Here's how the part is built. I have some questions about the finished solid (model axes, mm). Face numbers are marked on the shaded views. A direction names the side the tool comes from. Round coordinates to 2 decimals unless told otherwise and drop trailing zeros. Order: outer loops, then holes, each group sorted by start corner. A loop starts at its lowest first (then second) coordinate and runs counter-clockwise, first axis right, second up.
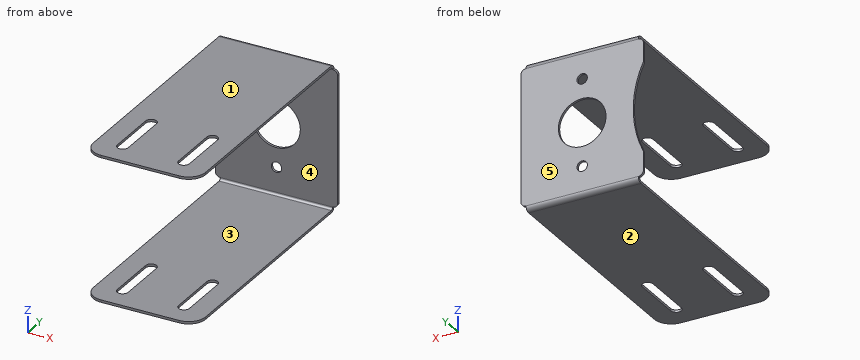
```python
from build123d import *

# Parameters (mm, degrees)
SKETCH1_W               = 36
SKETCH1_H               = 40
BASE_FLANGE1_DEPTH      = 0.7
EDGE_FLANGE1_DEPTH      = 33
EDGE_FLANGE1_BEND_DEPTH = 33
BREAK_CORNER1_START     = -0.7
BREAK_CORNER1_DEPTH     = 0.7
BREAK_CORNER2_START     = -21.4
BREAK_CORNER2_DEPTH     = 42.8
CUT_EXTRUDE1_DEPTH      = 78.892554201
CUT_EXTRUDE1_DEPTH_BACK = 78.892554201
CUT_EXTRUDE2_REACH      = 79.893
SKETCH11_R              = 7
SKETCH11_R_2            = 1.525
CUT_EXTRUDE3_REACH      = 79.893
SKETCH12_R              = 30


# Read off the part's stored shape, not the designer's step: Break-Corner1, Break-Corner2
# Sheet-metal steps are written as plain solids
with BuildPart() as part:
    # Sketch1 → Base-Flange1 (new body)
    with BuildSketch(Plane(origin=(0, 0, 0), x_dir=(1, 0, 0), z_dir=(0, 1, 0))):
        Rectangle(SKETCH1_W, SKETCH1_H)
    extrude(amount=-BASE_FLANGE1_DEPTH)

    # Edge-Flange1 section (across the edge) → Edge-Flange1 (add)
    with BuildSketch(Plane(origin=(16.5, -0.7, 20.7), x_dir=(0, 0, -1), z_dir=(-1, 0, 0))):
        with BuildLine():
            Line((-0.7, 0.7), (-0.7, 72))
            Line((-0.7, 72), (0, 72))
            Line((0, 72), (0, 0.7))
            ThreePointArc((0, 0.7), (0.205025253, 0.205025253), (0.7, 0))
            Line((0.7, 0), (0.7, -0.7))
            ThreePointArc((0.7, -0.7), (-0.289949494, -0.289949494), (-0.7, 0.7))
        make_face()
    extrude(amount=EDGE_FLANGE1_DEPTH)

    # Edge-Flange1 section 2 (across the edge) → Edge-Flange1 bend (add)
    with BuildSketch(Plane(origin=(-16.5, -0.7, -20.7), x_dir=(0, 0, 1), z_dir=(1, 0, 0))):
        with BuildLine():
            Line((-0.7, 0.7), (-0.7, 72))
            Line((-0.7, 72), (0, 72))
            Line((0, 72), (0, 0.7))
            ThreePointArc((0, 0.7), (0.205025253, 0.205025253), (0.7, 0))
            Line((0.7, 0), (0.7, -0.7))
            ThreePointArc((0.7, -0.7), (-0.289949494, -0.289949494), (-0.7, 0.7))
        make_face()
    extrude(amount=EDGE_FLANGE1_BEND_DEPTH)

    # Break-Corner1 outline → Break-Corner1 (cut)
    with BuildSketch(Plane(origin=(0, 0, 0), x_dir=(1, 0, 0), z_dir=(0, 1, 0)).offset(BREAK_CORNER1_START)):
        with BuildLine():
            Line((18, -20), (18, -18.5001))
            ThreePointArc((18, -18.5001), (17.560689461, -19.560689461), (16.5001, -20))
            Line((16.5001, -20), (18, -20))
        make_face()
        with BuildLine():
            ThreePointArc((16.5001, 20), (17.560689461, 19.560689461), (18, 18.5001))
            Line((18, 18.5001), (18, 20))
            Line((18, 20), (16.5001, 20))
        make_face()
        with BuildLine():
            ThreePointArc((-16.5001, -20), (-17.560689461, -19.560689461), (-18, -18.5001))
            Line((-18, -18.5001), (-18, -20))
            Line((-18, -20), (-16.5001, -20))
        make_face()
        with BuildLine():
            ThreePointArc((-18, 18.5001), (-17.560689461, 19.560689461), (-16.5001, 20))
            Line((-16.5001, 20), (-18, 20))
            Line((-18, 20), (-18, 18.5001))
        make_face()
    extrude(amount=BREAK_CORNER1_DEPTH, mode=Mode.SUBTRACT)

    # Break-Corner2 outline → Break-Corner2 (cut)
    with BuildSketch(Plane.XY.offset(BREAK_CORNER2_START)):
        with BuildLine():
            ThreePointArc((16.5, -67.7), (15.035533906, -71.235533906), (11.5, -72.7))
            Line((11.5, -72.7), (16.5, -72.7))
            Line((16.5, -72.7), (16.5, -67.7))
        make_face()
        with BuildLine():
            Line((-16.5, -72.7), (-11.5, -72.7))
            ThreePointArc((-11.5, -72.7), (-15.035533906, -71.235533906), (-16.5, -67.7))
            Line((-16.5, -67.7), (-16.5, -72.7))
        make_face()
    extrude(amount=BREAK_CORNER2_DEPTH, mode=Mode.SUBTRACT)

    # Sketch10 → Cut-Extrude1 (cut, two sides: drawn at the far end of the back side and taken through both)
    with BuildSketch(Plane.XY.offset(-CUT_EXTRUDE1_DEPTH_BACK)):
        with BuildLine():
            Line((-7.4, -50.7), (-7.4, -65.7))
            ThreePointArc((-7.4, -65.7), (-9, -67.3), (-10.6, -65.7))
            Line((-10.6, -65.7), (-10.6, -50.7))
            ThreePointArc((-10.6, -50.7), (-9, -49.1), (-7.4, -50.7))
        make_face()
        with BuildLine():
            Line((7.4, -50.7), (7.4, -65.7))
            ThreePointArc((7.4, -65.7), (9, -67.3), (10.6, -65.7))
            Line((10.6, -65.7), (10.6, -50.7))
            ThreePointArc((10.6, -50.7), (9, -49.1), (7.4, -50.7))
        make_face()
    extrude(amount=CUT_EXTRUDE1_DEPTH + CUT_EXTRUDE1_DEPTH_BACK, mode=Mode.SUBTRACT)

    # Sketch11 → Cut-Extrude2 (cut, up to next)
    with BuildSketch(Plane(origin=(0, 0, 0), x_dir=(1, 0, 0), z_dir=(0, 1, 0)), mode=Mode.PRIVATE) as cut_extrude2_sk1:
        with Locations(Location((0, 0, 0), (0, 0, 270))):
            Circle(SKETCH11_R)
    cut_extrude2_tool1 = extrude(cut_extrude2_sk1.sketch, amount=-CUT_EXTRUDE2_REACH, mode=Mode.PRIVATE) & part.part
    # Sketch11 → Cut-Extrude2 (cut, up to next)
    with BuildSketch(Plane(origin=(0, 0, 0), x_dir=(1, 0, 0), z_dir=(0, 1, 0)), mode=Mode.PRIVATE) as cut_extrude2_sk2:
        with Locations(Location((0, -12.7, 0), (0, 0, 270))):
            Circle(SKETCH11_R_2)
    cut_extrude2_tool2 = extrude(cut_extrude2_sk2.sketch, amount=-CUT_EXTRUDE2_REACH, mode=Mode.PRIVATE) & part.part
    # Sketch11 → Cut-Extrude2 (cut, up to next)
    with BuildSketch(Plane(origin=(0, 0, 0), x_dir=(1, 0, 0), z_dir=(0, 1, 0)), mode=Mode.PRIVATE) as cut_extrude2_sk3:
        with Locations(Location((0, 12.7, 0), (0, 0, 270))):
            Circle(SKETCH11_R_2)
    cut_extrude2_tool3 = extrude(cut_extrude2_sk3.sketch, amount=-CUT_EXTRUDE2_REACH, mode=Mode.PRIVATE) & part.part
    add(cut_extrude2_tool1.solids().sort_by_distance((0, 0, 0))[0], mode=Mode.SUBTRACT)
    add(cut_extrude2_tool2.solids().sort_by_distance((0, 0, 12.7))[0], mode=Mode.SUBTRACT)
    add(cut_extrude2_tool3.solids().sort_by_distance((0, 0, -12.7))[0], mode=Mode.SUBTRACT)

    # Sketch12 → Cut-Extrude3 (cut, up to next)
    with BuildSketch(Plane(origin=(0, 0, 0), x_dir=(1, 0, 0), z_dir=(0, 1, 0)), mode=Mode.PRIVATE) as cut_extrude3_sk1:
        with Locations((-45, 0)):
            Circle(SKETCH12_R)
    cut_extrude3_tool1 = extrude(cut_extrude3_sk1.sketch, amount=-CUT_EXTRUDE3_REACH, mode=Mode.PRIVATE) & part.part
    add(cut_extrude3_tool1.solids().sort_by_distance((-45, 0, 0))[0], mode=Mode.SUBTRACT)


solid = part.part
```
1. If we section it at C-C, the plane z = 0: Write out the boundary of the cut face in (x, y).
Evaluation:
outline: (-15, -0.7) - (-7, -0.7) - (-7, 0) - (-15, 0) - close; (7, -0.7) - (18, -0.7) - (18, 0) - (7, 0) - close
2. I'm going to push flat-ended pins straight in: P1, Ø0.8, axis at y = -54.5, z = -21, coming from the -X side; P2, Ø0.6, axis at y = -57.5, z = 21, coming from the +X side; P3, Ø11, axis at x = 0, z = 0, coming from the -Y side; P4, Ø4, axis at x = 10, z = 15.5, coming from the -Y side. Where does each tip first touch, or does it pass through?
Evaluation:
P1: stops at x = -16.5
P2: stops at x = 16.5
P3: passes through
P4: stops at y = -0.7
3. I need wall thicknesses on probe 1 along Z at (x, y) = (-5, -35.5); probe 2 along Y at (x, z) = (-13.5, -2.5); probe 3 along X at (y, z) = (-0.2, 12.7) (3 decimals). Which ranges of each line are inside material? Lowest first, please.
Evaluation:
probe 1: z = -21.4 to -20.7, 20.7 to 21.4
probe 2: y = -0.7 to 0
probe 3: x = -17.821 to -1.525, 1.525 to 18
4. If we section it at B-B, the plane y = -59: Write out the boundary of the cut face in (x, z), and give its area (3 significant figures).
Evaluation:
outline: (-16.5, -21.4) - (-10.6, -21.4) - (-10.6, -20.7) - (-16.5, -20.7) - close; (-16.5, 20.7) - (-10.6, 20.7) - (-10.6, 21.4) - (-16.5, 21.4) - close; (-7.4, -21.4) - (7.4, -21.4) - (7.4, -20.7) - (-7.4, -20.7) - close; (-7.4, 20.7) - (7.4, 20.7) - (7.4, 21.4) - (-7.4, 21.4) - close; (10.6, -21.4) - (16.5, -21.4) - (16.5, -20.7) - (10.6, -20.7) - close; (10.6, 20.7) - (16.5, 20.7) - (16.5, 21.4) - (10.6, 21.4) - close
area: 37.2 mm2
5. If we mould it in two halves opening along Z, with no side actions, what happens to the marked faces 1, 2 and 3? For each: released by +Z, released by -Z, zero draft, split by the parting line, or undercut.
Evaluation:
face 1: released by +Z
face 2: released by -Z
face 3: undercut
6. On a 3-axis mill with a long thin cutter (end or side, diameter ignored), from which of +Z, -Z, +X, -X, +Y, -Y can I reach the whole of each face in a straight line? I mean the marked faces 4 and 5. Say none if no direction works.
Evaluation:
face 4: +X, -X, -Y
face 5: +Z, -Z, +X, -X, +Y
7. If we section it at A-A, the plane x = -9: Write out the boundary of the cut face in (y, z), and give its area (3 significant figures).
Evaluation:
outline: (-72.7, -21.4) - (-67.3, -21.4) - (-67.3, -20.7) - (-72.7, -20.7) - close; (-72.7, 20.7) - (-67.3, 20.7) - (-67.3, 21.4) - (-72.7, 21.4) - close; (-49.1, -21.4) - (-1.4, -21.4) arc R1.4 ccw to (0, -20) - (0, 20) arc R1.4 ccw to (-1.4, 21.4) - (-49.1, 21.4) - (-49.1, 20.7) - (-1.4, 20.7) arc R0.7 cw to (-0.7, 20) - (-0.7, -20) arc R0.7 cw to (-1.4, -20.7) - (-49.1, -20.7) - close
area: 105 mm2
8. If we section it at D-D, the plane y = -32: Write out the boundary of the cut face in (x, z), and give its area (3 significant figures).
Evaluation:
outline: (-16.5, -21.4) - (16.5, -21.4) - (16.5, -20.7) - (-16.5, -20.7) - close; (-16.5, 20.7) - (16.5, 20.7) - (16.5, 21.4) - (-16.5, 21.4) - close
area: 46.2 mm2
